The listing builds one solid part. Answer for the finished solid, in the listing's coordinates (mm). Face numbers are marked on the shaded views. A direction names the side the tool comes from. Coordinates: 2 decimals unless noted, no trailing zeros. Order: outer loops, then holes, each group sorted by start corner. A loop starts at its lowest first (then second) coordinate and runs counter-clockwise, first axis right, second up. Notation, with made-up numbers: (-23.5, -21.75) -> (10.5, -21.75) arc R16 cw to (10.5, -2.75) -> close; hole circle Ø11 at (29.25, 53.25). An arc over 180 degrees is marked (long way). Return JSON: item names as keys, results as strings.
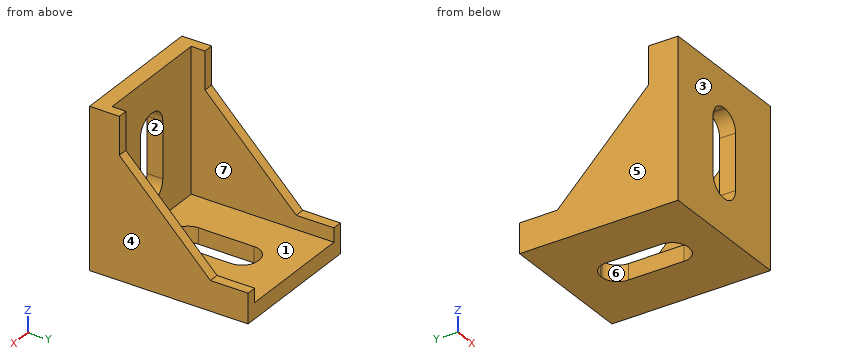
Autodesk Inventor part; units mm, degrees
ref_plane "YZ Plane" through (0, 0, 0) normal (1, 0, 0) x (0, 1, 0)
ref_plane "XZ Plane" through (0, 0, 0) normal (0, 1, 0) x (-1, 0, 0)
ref_plane "XY Plane" through (0, 0, 0) normal (0, 0, 1) x (1, 0, 0)
sketch "Sketch1" plane through (0, 0, 0) normal (0, 1, 0) x (-1, 0, 0)
  line L0 (0, 0) -> (17.5, 0)
  line L1 (17.5, 0) -> (17.5, -20)
  line L2 (17.5, -20) -> (-17.5, -20)
  line L3 (-17.5, -20) -> (-17.5, 20)
  line L4 (-17.5, 20) -> (17.5, 20)
  line L5 (17.5, 20) -> (17.5, 0)
  line L6 (15, -17.5) -> (15, 0)
  line L7 (15, 0) -> (15, 17.5)
  line L8 (15, 17.5) -> (-15, 17.5)
  line L9 (-15, 17.5) -> (-15, -17.5)
  line L10 (-15, -17.5) -> (15, -17.5)
  line L11 (0, 0) -> (0, 11)
  line L12 (0, 0) -> (0, -11)
  line L13 (0, 0) -> (4.25, 0)
  line L14 (4.25, 0) -> (4.25, -7)
  line L15 (0.25, -11) -> (-0.25, -11)
  line L16 (-4.25, -7) -> (-4.25, 7)
  line L17 (-0.25, 11) -> (0.25, 11)
  line L18 (4.25, 7) -> (4.25, 0)
  arc A0 (4.25, 7) -> (0.25, 11) centre (0.25, 7) ccw
  arc A1 (-0.25, 11) -> (-4.25, 7) centre (-0.25, 7) ccw
  arc A2 (0.25, -11) -> (4.25, -7) centre (0.25, -7) ccw
  arc A3 (-4.25, -7) -> (-0.25, -11) centre (-0.25, -7) ccw
  point P0 (4.25, -11)
  point P1 (-4.25, -11)
  point P2 (4.25, 11)
  dimension "d2" = 17.5
  dimension "d3" = 20
  dimension "d4" = 35
  dimension "d5" = 40
  dimension "d6" = 35
  dimension "d7" = 2.5
  dimension "d8" = 11
  dimension "d9" = 11
  dimension "d10" = 4.25
  dimension "d11" = 8.5
  dimension "d12" = 4
extrude "Extrusion1" add sketch "Sketch1" along normal blind 4 contours L6 L10 L9 L8 L7 | L1 L2 L3 L4 L5
sketch "Sketch2" plane through (0, 4, 0) normal (0, 1, 0) x (1, 0, 0)
  line L0 (-17.5, -20) -> (17.5, -20)
  line L1 (17.5, -20) -> (17.5, 20)
  line L2 (17.5, 20) -> (-17.5, 20)
  line L3 (-17.5, 20) -> (-17.5, -20)
  line L4 (-4.25, -7) -> (-4.25, 7)
  arc A0 (-0.25, 11) -> (-4.25, 7) centre (-0.25, 7) ccw
  line L5 (-0.25, 11) -> (0.25, 11)
  arc A1 (4.25, 7) -> (0.25, 11) centre (0.25, 7) ccw
  line L6 (4.25, 7) -> (4.25, -7)
  arc A2 (0.25, -11) -> (4.25, -7) centre (0.25, -7) ccw
  line L7 (0.25, -11) -> (-0.25, -11)
  arc A3 (-4.25, -7) -> (-0.25, -11) centre (-0.25, -7) ccw
  line L8 (-17.5, 20) -> (-17.5, -20)
  line L9 (-17.5, 20) -> (-17.5, 16)
  line L10 (-17.5, 16) -> (17.5, 16)
  line L11 (17.5, -20) -> (17.5, 20)
  point P0 (0, 0)
  dimension "d15" = 4
extrude "Extrusion2" add sketch "Sketch2" along normal blind 36 contours L3 L2 L1 L10
sketch "Sketch3" plane through (17.5, 0, -20) normal (0, 0, -1) x (-1, 0, 0)
  line L0 (0, 0) -> (35, 0)
  line L1 (35, 0) -> (35, 40)
  line L2 (0, 40) -> (35, 40)
  line L3 (0, 0) -> (0, 40)
  line L4 (17.5, 0) -> (17.5, 40)
  line L5 (35, 40) -> (0, 40)
  line L6 (17.5, 20) -> (17.5, 9)
  line L7 (17.5, 20) -> (17.5, 31)
  line L8 (17.5, 31) -> (17.25, 31)
  line L9 (13.25, 27) -> (13.25, 13)
  line L10 (17.25, 9) -> (17.75, 9)
  line L11 (21.75, 13) -> (21.75, 27)
  line L12 (17.75, 31) -> (17.5, 31)
  arc A0 (13.25, 13) -> (17.25, 9) centre (17.25, 13) ccw
  arc A1 (17.75, 9) -> (21.75, 13) centre (17.75, 13) ccw
  arc A2 (17.25, 31) -> (13.25, 27) centre (17.25, 27) ccw
  arc A3 (21.75, 27) -> (17.75, 31) centre (17.75, 27) ccw
  point P0 (13.25, 31)
  point P1 (13.25, 9)
  point P2 (21.75, 9)
  point P3 (21.75, 31)
  dimension "d18" = 11
  dimension "d19" = 11
  dimension "d20" = 4.25
  dimension "d21" = 22
  dimension "d22" = 8.5
  dimension "d23" = 4
extrude "Extrusion3" cut sketch "Sketch3" against normal blind 4 contours L10 A0 L9 A2 L8 L4 | L4 L12 A3 L11 A1 L10
sketch "Sketch4" plane through (17.5, 0, 20) normal (1, 0, 0) x (0, 0, -1)
  line L0 (0, 0) -> (40, 0)
  line L1 (40, 0) -> (40, 40)
  line L2 (36, 40) -> (40, 40)
  line L3 (36, 4) -> (36, 40)
  line L4 (0, 4) -> (36, 4)
  line L5 (0, 0) -> (0, 4)
  line L6 (36, 4) -> (0, 4)
  line L7 (0, 4) -> (0, 7.5)
  line L8 (0, 7.5) -> (9.5, 7.5)
  line L9 (36, 4) -> (36, 40)
  line L10 (36, 40) -> (32.5, 40)
  line L11 (32.5, 40) -> (32.5, 30.5)
  line L12 (0, 7.5) -> (9.5, 7.5)
  line L13 (32.5, 40) -> (32.5, 30.5)
  line L14 (32.5, 30.5) -> (9.5, 7.5)
  point P0 (20, 0)
  dimension "d26" = 3.5
  dimension "d27" = 3.5
  dimension "d28" = 9.5
  dimension "d29" = 9.5
extrude "Extrusion4" add sketch "Sketch4" against normal blind 2.5 contours L7 L8 L14 L11 L10 L3 L4
mirror "Mirror1" about plane through (0, 0, 0) normal (1, 0, 0) of "Extrusion4"
ref_plane "Work Plane1" through (0, 0, 0) normal (1, 0, 0) x (0, 1, 0)
properties part number "KE HOC NHOM DINH HINH"
1. Consider line 1 (X direction, y = 26.5, z = -17); line 2 (X direction, y = 24.5, z = -8); line 3 (Y direction, x = 13.5, z = 13). Determine where each line is inside the solid, lowest interval first. Write a range as from..to.
Answer block:
{"line 1": "x = -17.5..-4.25, 4.25..17.5", "line 2": "x = -17.5..-15, 15..17.5", "line 3": "y = 0..4"}
2. Each of these flat-tipped pins is pushed along its axis until it touches: pin 1 Ø0.8 at (x, y) = (-16.5, 37.5) entering from +Z; pin 2 Ø0.8 at (x, z) = (-16, 13.5) entering from +Y; pin 3 Ø9 at (x, y) = (-3, 30.5) entering from +Z. Where does it stop, or does it pass through?
Answer block:
{"pin 1": "stops at z = -12.5", "pin 2": "stops at y = 7.5", "pin 3": "stops at z = -16"}
3. The part is cut by section B-B on z = 5. Give the vertices of the cut face in (x, y), and give its area (3 significant figures).
Answer block:
{"outline": "(-17.5, 0) -> (-4.25, 0) -> (-4.25, 4) -> (-15, 4) -> (-15, 13) -> (-17.5, 13) -> close; (4.25, 0) -> (17.5, 0) -> (17.5, 13) -> (15, 13) -> (15, 4) -> (4.25, 4) -> close", "area": "151 mm2"}
4. The part is cut by section A-A on y = 16. Give the vertices of the cut face in (x, z).
Answer block:
{"outline": "(-17.5, -20) -> (-4.25, -20) -> (-4.25, -16) -> (-15, -16) -> (-15, 2) -> (-17.5, 2) -> close; (4.25, -20) -> (17.5, -20) -> (17.5, 2) -> (15, 2) -> (15, -16) -> (4.25, -16) -> close"}
5. The part is cut by section C-C on x = -2. Give the vertices of the cut face in (y, z), and give its area (3 significant figures).
Answer block:
{"outline": "(0, -20) -> (9.4, -20) -> (9.4, -16) -> (4, -16) -> (4, -10.6) -> (0, -10.6) -> close; (0, 10.6) -> (4, 10.6) -> (4, 20) -> (0, 20) -> close; (30.6, -20) -> (40, -20) -> (40, -16) -> (30.6, -16) -> close", "area": "134 mm2"}
6. The part is cut by section D-D on z = -17. Give the vertices of the cut face in (x, y).
Answer block:
{"outline": "(-17.5, 0) -> (17.5, 0) -> (17.5, 40) -> (-17.5, 40) -> close; hole (-4.25, 13) arc R4 ccw to (-0.25, 9) -> (0.25, 9) arc R4 ccw to (4.25, 13) -> (4.25, 27) arc R4 ccw to (0.25, 31) -> (-0.25, 31) arc R4 ccw to (-4.25, 27) -> close"}
7. Determine the mould class of the marked faces 4, 5, 6 and 7 for opening direction X: pulls with the +X half, pulls with the -X half, needs draft (parallel to the pull), parting line crosses it, or undercut.
Answer block:
{"face 4": "pulls with the +X half", "face 5": "pulls with the -X half", "face 6": "undercut", "face 7": "undercut"}
8. For the marked faces 1, 2 and 3, determine the directions among +Z, -Z, +X, -X, +Y, -Y from which every point of the face is accessible in a straight line to the end or side of a thin tool.
Answer block:
{"face 1": "+Z, +Y", "face 2": "+Y, -Y", "face 3": "+Z, -Z, +X, -X, -Y"}
